```python
from build123d import *

# Parameters (mm, degrees)
BOSS_EXTRUDE1_DEPTH  = 2
SKETCH2_W            = 2
SKETCH2_H            = 26
BOSS_EXTRUDE2_DEPTH  = 24
BOSS_EXTRUDE3_DEPTH  = 2
SKETCH4_R            = 4
CUT_EXTRUDE1_DEPTH   = 2
BOSS_EXTRUDE4_DEPTH  = 26
CUT_EXTRUDE2_DEPTH   = 26
BOSS_EXTRUDE5_DEPTH  = 2
SKETCH8_R            = 7.515013345
SKETCH8_R_2          = 4.48835621
BOSS_EXTRUDE6_DEPTH  = 4
SKETCH9_R            = 3.1
CUT_EXTRUDE3_DEPTH   = 10
SKETCH10_R           = 4
CUT_EXTRUDE4_DEPTH   = 10
SKETCH11_R           = 4
SKETCH11_R_2         = 3.1
BOSS_EXTRUDE7_DEPTH  = 7
SKETCH12_R           = 4
BOSS_EXTRUDE8_DEPTH  = 1
SKETCH13_W           = 5
SKETCH13_H           = 10
CUT_EXTRUDE5_DEPTH   = 10
SKETCH14_W           = 5
SKETCH14_H           = 10
CUT_EXTRUDE6_DEPTH   = 4
SKETCH15_W           = 5
SKETCH15_H           = 10
BOSS_EXTRUDE9_DEPTH  = 2
SKETCH16_W           = 5
SKETCH16_H           = 2
BOSS_EXTRUDE10_DEPTH = 2
SKETCH17_W           = 5
SKETCH17_H           = 14
BOSS_EXTRUDE11_DEPTH = 2
FILLET1_R            = 10


with BuildPart() as part:
    # Sketch1 → Boss-Extrude1 (new body)
    with BuildSketch(Plane(origin=(0, 0, 0), x_dir=(1, 0, 0), z_dir=(0, 1, 0))):
        with BuildLine():
            Line((40, 13), (0, 13))
            ThreePointArc((0, 13), (-13, 0), (0, -13))
            Line((0, -13), (40, -13))
            Line((40, -13), (40, 13))
        make_face()
    extrude(amount=BOSS_EXTRUDE1_DEPTH)

    # Sketch2 → Boss-Extrude2 (add)
    with BuildSketch(Plane(origin=(0, 2, 0), x_dir=(1, 0, 0), z_dir=(0, 1, 0))):
        with Locations((39, 0)):
            Rectangle(SKETCH2_W, SKETCH2_H)
    extrude(amount=BOSS_EXTRUDE2_DEPTH)

    # Sketch3 → Boss-Extrude3 (add)
    with BuildSketch(Plane(origin=(0, 26, 0), x_dir=(1, 0, 0), z_dir=(0, 1, 0))):
        with BuildLine():
            Line((40, -13), (0, -13))
            ThreePointArc((0, -13), (-13, 0), (0, 13))
            Line((0, 13), (40, 13))
            Line((40, 13), (40, -13))
        make_face()
    extrude(amount=BOSS_EXTRUDE3_DEPTH)

    # Sketch4 → Cut-Extrude1 (cut)
    with BuildSketch(Plane(origin=(40, 0, 0), x_dir=(0, 0, -1), z_dir=(1, 0, 0))):
        with Locations((0, 14)):
            Circle(SKETCH4_R)
    extrude(amount=-CUT_EXTRUDE1_DEPTH, mode=Mode.SUBTRACT)

    # Sketch5 → Boss-Extrude4 (add)
    with BuildSketch(Plane.XY.offset(13)):
        Polygon((38, 5), (34, 2), (31.333333333, 0), (31.333333333, 2), (40, 8.5), (40, 6.5), align=None)
        Polygon((40, 21.5), (38, 23), (34, 26), (31.333333333, 28), (31.333333333, 26), (40, 19.5), align=None)
    extrude(amount=-BOSS_EXTRUDE4_DEPTH)

    # Sketch6 → Cut-Extrude2 (cut)
    with BuildSketch(Plane.XY.offset(13)):
        Polygon((38, 5), (31.333333333, 0), (40, 0), (40, 6.5), align=None)
        Polygon((40, 28), (40, 21.5), (38, 23), (31.333333333, 28), align=None)
    extrude(amount=-CUT_EXTRUDE2_DEPTH, mode=Mode.SUBTRACT)

    # Sketch7 → Boss-Extrude5 (add)
    with BuildSketch(Plane.XY.offset(13)):
        Polygon((40, 21.5), (31.333333333, 28), (20.333333333, 28), (20.333333333, 0), (31.333333333, 0), (40, 6.5), align=None)
    boss_extrude5 = extrude(amount=BOSS_EXTRUDE5_DEPTH)

    # Mirror1: Boss-Extrude5 across plane
    add(boss_extrude5.mirror(Plane.XY))

    # Sketch8 → Boss-Extrude6 (add)
    with BuildSketch(Plane.ZY.offset(-38)):
        with Locations(Location((0, 14, 0), (0, 0, 111.335065793))):
            Circle(SKETCH8_R)
        with Locations((0, 14)):
            Circle(SKETCH8_R_2, mode=Mode.SUBTRACT)
    extrude(amount=BOSS_EXTRUDE6_DEPTH)

    # Sketch9 → Cut-Extrude3 (cut)
    with BuildSketch(Plane.XZ):
        with Locations(Location((0, 0, 0), (0, 0, 270))):
            Circle(SKETCH9_R)
    extrude(amount=-CUT_EXTRUDE3_DEPTH, mode=Mode.SUBTRACT)

    # Sketch10 → Cut-Extrude4 (cut)
    with BuildSketch(Plane(origin=(0, 28, 0), x_dir=(1, 0, 0), z_dir=(0, 1, 0))):
        with Locations(Location((0, 0, 0), (0, 0, 270))):
            Circle(SKETCH10_R)
    extrude(amount=-CUT_EXTRUDE4_DEPTH, mode=Mode.SUBTRACT)

    # Sketch11 → Boss-Extrude7 (add)
    with BuildSketch(Plane.XZ):
        with Locations(Location((0, 0, 0), (0, 0, 90))):
            Circle(SKETCH11_R)
        with Locations(Location((0, 0, 0), (0, 0, 270))):
            Circle(SKETCH11_R_2, mode=Mode.SUBTRACT)
    extrude(amount=BOSS_EXTRUDE7_DEPTH)

    # Sketch12 → Boss-Extrude8 (add)
    with BuildSketch(Plane.XZ.offset(7)):
        with Locations(Location((0, 0, 0), (0, 0, 90))):
            Circle(SKETCH12_R)
    extrude(amount=BOSS_EXTRUDE8_DEPTH)

    # Sketch13 → Cut-Extrude5 (cut)
    with BuildSketch(Plane.XY.offset(15)):
        with Locations((27.833333333, 14)):
            Rectangle(SKETCH13_W, SKETCH13_H)
    extrude(amount=-CUT_EXTRUDE5_DEPTH, mode=Mode.SUBTRACT)

    # Sketch14 → Cut-Extrude6 (cut)
    with BuildSketch(Plane(origin=(0, 0, -15), x_dir=(-1, 0, 0), z_dir=(0, 0, -1))):
        with Locations((-27.833333333, 14)):
            Rectangle(SKETCH14_W, SKETCH14_H)
    extrude(amount=-CUT_EXTRUDE6_DEPTH, mode=Mode.SUBTRACT)

    # Sketch15 → Boss-Extrude9 (add)
    with BuildSketch(Plane.XY.offset(15)):
        with Locations((27.833333333, 14)):
            Rectangle(SKETCH15_W, SKETCH15_H)
    extrude(amount=-BOSS_EXTRUDE9_DEPTH)

    # Sketch16 → Boss-Extrude10 (add)
    with BuildSketch(Plane(origin=(0, 0, -15), x_dir=(-1, 0, 0), z_dir=(0, 0, -1))):
        with Locations((-27.833333333, 20)):
            Rectangle(SKETCH16_W, SKETCH16_H)
        with Locations((-27.833333333, 8)):
            Rectangle(SKETCH16_W, SKETCH16_H)
    extrude(amount=BOSS_EXTRUDE10_DEPTH)

    # Sketch17 → Boss-Extrude11 (add)
    with BuildSketch(Plane(origin=(0, 0, -17), x_dir=(-1, 0, 0), z_dir=(0, 0, -1))):
        with Locations((-27.833333333, 14)):
            Rectangle(SKETCH17_W, SKETCH17_H)
    extrude(amount=BOSS_EXTRUDE11_DEPTH)

    # Fillet1
    # the kernel refuses this fillet: 10 mm, written as the material it adds along each edge
    with BuildSketch(Plane(origin=(20.333333333, 28, 13), x_dir=(0, 0, 1), z_dir=(0, -1, 0))) as fillet1_piece_1:
        with BuildLine():
            CenterArc((10, 6), FILLET1_R, 180, 36.869897646)
            Line((0, 6), (0, 0))
            Line((0, 0), (2, 0))
        make_face()
    extrude(amount=2)
    with BuildSketch(Plane(origin=(20.333333333, 2, 13), x_dir=(-1, 0, 0), z_dir=(0, -1, 0))) as fillet1_piece_2:
        with BuildLine():
            CenterArc((6, -10), FILLET1_R, 90, 36.869897646)
            Line((0, -2), (0, 0))
            Line((0, 0), (6, 0))
        make_face()
    extrude(amount=2)
    with BuildSketch(Plane(origin=(20.333333333, 2, -13), x_dir=(-1, 0, 0), z_dir=(0, -1, 0))) as fillet1_piece_3:
        with BuildLine():
            CenterArc((6, 10), FILLET1_R, 233.130102354, 36.869897646)
            Line((0, 2), (0, 0))
            Line((0, 0), (6, 0))
        make_face()
    extrude(amount=2)
    with BuildSketch(Plane(origin=(20.333333333, 28, -13), x_dir=(0, 0, -1), z_dir=(0, -1, 0))) as fillet1_piece_4:
        with BuildLine():
            CenterArc((10, -6), FILLET1_R, 143.130102354, 36.869897646)
            Line((0, -6), (0, 0))
            Line((0, 0), (2, 0))
        make_face()
    extrude(amount=2)


solid = part.part
```
Design review of the part built by this model. Coordinates are the model's own, in mm. A direction names the side the tool comes from. Round coordinates to 2 decimals unless told otherwise and drop trailing zeros. Write each loop counter-clockwise with the first axis right and the second up, starting at its lowest first coordinate (ties: lowest second). Pieces come first, ordered by that corner, then holes.
Item 1: For probe 1 along Z at (x, y) = (25, 4.5); probe 2 along Y at (x, z) = (13.5, 1); probe 3 along Y at (x, z) = (36.85, 0), list the stretches that pass through material, from the lowest coordinate up.
Item 2: We need section A-A on y = 14. Write out the cut boundary in (x, z), and give its area (3 significant figures).
Item 3: We need section D-D on x = 32. Write out the cut boundary in (y, z), and give its area (3 significant figures).
Item 4: We need section C-C on z = 9. Write out the cut boundary in (x, y), and give its area (3 significant figures).
Item 5: The part is to be moulded in two halves that separate along Z. For faces 1 (the flat face through (40, 17, 4)), 2 (the flat face through (9, 26, 0)), 3 (the flat face through (7, 1, 13)), say which applies: +Z half, -Z half, draft (parallel to the pull), parting line (faces both ways), or undercut.
Item 6: Clearance check with flat-ended pins moving along their axes: pin 1 Ø2 at (y, z) = (9.5, 13.5) entering from -X; pin 2 Ø1 at (x, y) = (10, 27.5) entering from +Z; pin 3 Ø2 at (x, y) = (6.5, 1) entering from -Z. State where each tip first meets the part, or that it passes through.
Item 7: We need section B-B on x = 24. Write out the cut boundary in (y, z), and give its area (3 significant figures).
Item 8: For faces 4 (the flat face through (34.62, 23.535, 0.182)), 5 (the flat face through (25.333, 14, -18)), 6 (the flat face through (28, 7, -17)), 7 (the flat face through (25.333, 14, -14)), 8 (the flat face through (0, -7, 0)), list the 3-axis set-ups (+Z, -Z, +X, -X, +Y, -Y) from which the entire face can be reached by the end or side of a thin tool; tool diameter is ignored.
Returned:
1. probe 1: z = -15 to -13, 13 to 15
1. probe 2: y = 0 to 2, 26 to 28
1. probe 3: y = 4.14 to 6.14, 6.48 to 9.51, 18.49 to 21.52, 21.86 to 23.86
2. outline: (20.33, -15) - (25.33, -15) - (25.33, -13) - (20.33, -13) - close; (20.33, 13) - (38, 13) - (38, 7.52) - (34, 7.52) - (34, 4.49) - (38, 4.49) - (38, 4) - (40, 4) - (40, 15) - (20.33, 15) - close; (25.33, -19) - (30.33, -19) - (30.33, -17) - (25.33, -17) - close; (30.33, -15) - (40, -15) - (40, -4) - (38, -4) - (38, -4.49) - (34, -4.49) - (34, -7.52) - (38, -7.52) - (38, -13) - (30.33, -13) - close
2. area: 139 mm2
3. outline: (0.5, -15) - (27.5, -15) - (27.5, 15) - (0.5, 15) - close; hole (2.5, -13) - (25.5, -13) - (25.5, 13) - (2.5, 13) - close
3. area: 212 mm2
4. outline: (-9.38, 0) - (31.33, 0) - (40, 6.5) - (40, 21.5) - (31.33, 28) - (-9.38, 28) - (-9.38, 26) - (31.33, 26) - (38, 21) - (38, 7) - (31.33, 2) - (-9.38, 2) - close
4. area: 223 mm2
5. face 1: draft
5. face 2: undercut
5. face 3: +Z half
6. pin 1: stops at x = 20.33
6. pin 2: stops at z = 13
6. pin 3: stops at z = -13
7. outline: (0, -15) - (28, -15) - (28, 15) - (0, 15) - close; hole (2, -13) - (26, -13) - (26, 13) - (2, 13) - close
7. area: 216 mm2
8. face 4: -X
8. face 5: -Z, -X, +Y, -Y
8. face 6: -Z, +X, -X, -Y
8. face 7: none
8. face 8: +Y
